The listing builds one solid part. Answer for the finished solid, in the listing's coordinates (mm). A direction names the side the tool comes from. Round coordinates to 2 decimals unless told otherwise and drop trailing zeros. Order: outer loops, then holes, each group sorted by start corner. A loop starts at its lowest first (then second) coordinate and runs counter-clockwise, first axis right, second up. Notation, with made-up numbers: M -4,73.25 L 1,73.25 A20 ccw 1,102.25 Z; hole C -28,7 d3. An arc over 180 degrees is marked long. Put each result on its own line as item: value. Start each with the question number.
1. The part is cut by section B-B (z = 49). Give the vertices of the cut face in (x, y) (3 decimals), then the cut area to 3 significant figures.
2. The mould has two halves that part along Z. Classify faces 1 (the face through (10, 14, 29.667)), 2 (the face through (10, 14, 4.648)), 3 (the face through (9.525, 14.7, 49.4)): +Z half, -Z half, draft (parallel to the pull), parting line (faces both ways), or undercut.
3. Each of these flat-tipped pins is pushed along its axis until it touches: pin 1 Ø5.5 at (x, z) = (6.5, 49) entering from -Y; pin 2 Ø5.5 at (x, z) = (6.5, 49) entering from +Y; pin 3 Ø0.6 at (x, z) = (6.5, 51.5) entering from -Y; pin 4 Ø2 at (x, y) = (9, 9.5) entering from +Z. Where does it stop, or does it pass through?
4. The part is cut by section C-C (x = 15). Give the vertices of the cut face in (y, z), then the cut area to 3 significant figures.
5. The part is cut by section A-A (y = 8.5). Give the vertices of the cut face in (x, z).
6. The part is cut by section D-D (z = 5.5). Give the vertices of the cut face in (x, y).
7. Consider line 1 (Y direction, x = 5.75, z = 47.5); line 2 (X direction, y = 6.25, z = 26.5); line 3 (Y direction, x = 6, z = 10.5). Determine where each line is inside the solid, lowest interval first.
8. Which of the six approach directions +Z, -Z, +X, -X, +Y, -Y give full straight-line access (tool end or side, diameter ignored) to faces 4 (the face through (6, 15.621, 49)), 5 (the face through (6, 14, 46.66)), 6 (the face through (2.464, 6, 25)), 7 (the face through (17.704, 14, 17)), 8 (the face through (6, 15.367, 50))?
from build123d import *

# Parameters (mm, degrees)
BOSS_EXTRUDE1_DEPTH      = 50.9778
CHAMFER1_SIZE            = 0.889
CHAMFER1_SIZE2           = 1.269623578
BOSS_EXTRUDE2_DEPTH      = 1.27
BOSS_EXTRUDE2_DEPTH_BACK = 4.318
CUT_EXTRUDE1_DEPTH       = 5.08
SKETCH4_W                = 3.175
SKETCH4_H                = 1.5875
BOSS_EXTRUDE3_DEPTH      = 0.762
SKETCH5_W                = 15.24
SKETCH5_H                = 25.019
BOSS_EXTRUDE4_DEPTH      = 2.9972


with BuildPart() as part:
    # Sketch1 → Boss-Extrude1 (new body)
    with BuildSketch(Plane.XY):
        Polygon((0, 0), (2.4638, 0), (2.4638, 11.303), (17.7038, 11.303), (17.7038, 0), (20.1676, 0), (20.1676, 12.954), (0, 12.954), align=None)
    extrude(amount=BOSS_EXTRUDE1_DEPTH)

    # Chamfer1
    chamfer1_edges = [part.edges().sort_by_distance(p)[0] for p in [
        (0, 6.477, 0),
        (20.1676, 6.477, 0),
    ]]
    chamfer1_side = [part.faces().sort_by_distance(p)[0] for p in [
        (1.2319, 0.239695266, 0),
    ]]
    chamfer(chamfer1_edges, length=CHAMFER1_SIZE, length2=CHAMFER1_SIZE2, reference=chamfer1_side[0])

    # Sketch2 → Boss-Extrude2 (add, two sides: drawn at the far end of the back side and taken through both)
    with BuildSketch(Plane.XY.offset(50.9778).offset(-BOSS_EXTRUDE2_DEPTH_BACK)):
        with BuildLine():
            Line((3.048, 12.954), (8.255, 12.954))
            ThreePointArc((8.255, 12.954), (9.153025612, 13.325974388), (9.525, 14.224))
            Line((9.525, 14.224), (9.525, 15.113))
            ThreePointArc((9.525, 15.113), (9.376210245, 15.472210245), (9.017, 15.621))
            Line((9.017, 15.621), (2.286, 15.621))
            ThreePointArc((2.286, 15.621), (1.926789755, 15.472210245), (1.778, 15.113))
            Line((1.778, 15.113), (1.778, 14.224))
            ThreePointArc((1.778, 14.224), (2.149974388, 13.325974388), (3.048, 12.954))
        make_face()
    extrude(amount=BOSS_EXTRUDE2_DEPTH + BOSS_EXTRUDE2_DEPTH_BACK)

    # Sketch3 → Cut-Extrude1 (cut)
    with BuildSketch(Plane.XY.offset(52.2478)):
        with BuildLine():
            Line((9.271, 14.224), (9.271, 15.113))
            ThreePointArc((9.271, 15.113), (9.196605122, 15.292605122), (9.017, 15.367))
            Line((9.017, 15.367), (2.286, 15.367))
            ThreePointArc((2.286, 15.367), (2.106394878, 15.292605122), (2.032, 15.113))
            Line((2.032, 15.113), (2.032, 14.224))
            ThreePointArc((2.032, 14.224), (2.32957951, 13.50557951), (3.048, 13.208))
            Line((3.048, 13.208), (8.255, 13.208))
            ThreePointArc((8.255, 13.208), (8.97342049, 13.50557951), (9.271, 14.224))
        make_face()
    extrude(amount=-CUT_EXTRUDE1_DEPTH, mode=Mode.SUBTRACT)

    # Sketch4 → Boss-Extrude3 (add)
    with BuildSketch(Plane(origin=(0, 12.954, 0), x_dir=(1, 0, 0), z_dir=(0, 1, 0))):
        with Locations((10.0838, -34.43605)):
            Rectangle(SKETCH4_W, SKETCH4_H)
    extrude(amount=BOSS_EXTRUDE3_DEPTH)

    # Sketch5 → Boss-Extrude4 (add)
    with BuildSketch(Plane(origin=(0, 12.954, 0), x_dir=(1, 0, 0), z_dir=(0, 1, 0))):
        with Locations((10.0838, -17.1577)):
            Rectangle(SKETCH5_W, SKETCH5_H)
    extrude(amount=BOSS_EXTRUDE4_DEPTH)


solid = part.part
Resolved:
1. outline: M 0,0 L 2.464,0 L 2.464,11.303 L 17.704,11.303 L 17.704,0 L 20.168,0 L 20.168,12.954 L 8.255,12.954 A1.27 ccw 9.525,14.224 L 9.525,15.113 A0.508 ccw 9.017,15.621 L 2.286,15.621 A0.508 ccw 1.778,15.113 L 1.778,14.224 A1.27 ccw 3.048,12.954 L 0,12.954 Z; hole M 2.032,14.224 A1.016 ccw 3.048,13.208 L 8.255,13.208 A1.016 ccw 9.271,14.224 L 9.271,15.113 A0.254 ccw 9.017,15.367 L 2.286,15.367 A0.254 ccw 2.032,15.113 Z
1. area: 93.7 mm2
2. face 1: undercut
2. face 2: -Z half
2. face 3: draft
3. pin 1: y = 11.3
3. pin 2: y = 15.62
3. pin 3: y = 12.95
3. pin 4: through
4. outline: M 11.3,0 L 12.95,0 L 12.95,4.65 L 15.95,4.65 L 15.95,29.67 L 12.95,29.67 L 12.95,50.98 L 11.3,50.98 Z
4. area: 159 mm2
5. outline: M 0,1.27 L 0.89,0 L 2.46,0 L 2.46,50.98 L 0,50.98 Z; M 17.7,0 L 19.28,0 L 20.17,1.27 L 20.17,50.98 L 17.7,50.98 Z
6. outline: M 0,0 L 2.46,0 L 2.46,11.3 L 17.7,11.3 L 17.7,0 L 20.17,0 L 20.17,12.95 L 17.7,12.95 L 17.7,15.95 L 2.46,15.95 L 2.46,12.95 L 0,12.95 Z
7. line 1: 11.3 to 13.21, 15.37 to 15.62
7. line 2: 0 to 2.46, 17.7 to 20.17
7. line 3: 11.3 to 15.95
8. face 4: +Z, +X, -X, +Y
8. face 5: +X, -X, +Y
8. face 6: +Z, -Z, -Y
8. face 7: +Z, -Z, +X, +Y
8. face 8: +Z
